```python
from build123d import *

# Parameters (mm, degrees)
SKETCH1_W           = 65.079845806
SKETCH1_H           = 55
SKETCH1_R           = 4
BOSS_EXTRUDE1_DEPTH = 3
SKETCH2_R           = 1
CUT_EXTRUDE1_DEPTH  = 3
FILLET1_R           = 0.5
SKETCH3_R           = 1
CUT_EXTRUDE2_DEPTH  = 52.961426281


with BuildPart() as part:
    # Sketch1 → Boss-Extrude1 (new body)
    with BuildSketch(Plane(origin=(0, 548.352995908, 0), x_dir=(1, 0, 0), z_dir=(0, 1, 0))):
        with Locations((-11.445754552, 0)):
            Rectangle(SKETCH1_W, SKETCH1_H)
        with Locations(Location((0, 0, 0), (0, 0, 270))):
            Circle(SKETCH1_R, mode=Mode.SUBTRACT)
    extrude(amount=BOSS_EXTRUDE1_DEPTH)

    # Sketch2 → Cut-Extrude1 (cut)
    with BuildSketch(Plane(origin=(0, 551.352995908, 0), x_dir=(1, 0, 0), z_dir=(0, 1, 0))):
        with Locations(Location((0, 8, 0), (0, 0, 270))):
            Circle(SKETCH2_R)
        with Locations(Location((5.656854249, 5.656854249, 0), (0, 0, 270))):
            Circle(SKETCH2_R)
        with Locations(Location((8, 0, 0), (0, 0, 270))):
            Circle(SKETCH2_R)
        with Locations(Location((5.656854249, -5.656854249, 0), (0, 0, 270))):
            Circle(SKETCH2_R)
        with Locations(Location((0, -8, 0), (0, 0, 270))):
            Circle(SKETCH2_R)
        with Locations(Location((-5.656854249, -5.656854249, 0), (0, 0, 270))):
            Circle(SKETCH2_R)
        with Locations(Location((-8, 0, 0), (0, 0, 270))):
            Circle(SKETCH2_R)
        with Locations(Location((-5.656854249, 5.656854249, 0), (0, 0, 270))):
            Circle(SKETCH2_R)
    extrude(amount=-CUT_EXTRUDE1_DEPTH, mode=Mode.SUBTRACT)

    # Fillet1
    fillet1_edges = [part.edges().sort_by_distance(p)[0] for p in [
        (21.094168351, 551.352995908, 0),
        (-11.445754552, 551.352995908, -27.5),
        (-43.985677455, 551.352995908, 0),
        (-11.445754552, 548.352995908, -27.5),
        (21.094168351, 548.352995908, 0),
        (-11.445754552, 548.352995908, 27.5),
        (-43.985677455, 548.352995908, 0),
        (-43.985677455, 549.852995908, -27.5),
        (21.094168351, 549.852995908, -27.5),
        (21.094168351, 549.852995908, 27.5),
        (-43.985677455, 549.852995908, 27.5),
        (-11.445754552, 551.352995908, 27.5),
    ]]
    fillet(fillet1_edges, radius=FILLET1_R)

    # Sketch3 → Cut-Extrude2 (cut, through all)
    with BuildSketch(Plane(origin=(0, 551.352995908, 0), x_dir=(1, 0, 0), z_dir=(0, 1, 0))):
        with Locations(Location((-33.485677455, -24, 0), (0, 0, 270))):
            Circle(SKETCH3_R)
        with Locations(Location((-23.485677455, -24, 0), (0, 0, 270))):
            Circle(SKETCH3_R)
        with Locations(Location((16.514322545, -12, 0), (0, 0, 270))):
            Circle(SKETCH3_R)
        with Locations(Location((16.514322545, 12, 0), (0, 0, 270))):
            Circle(SKETCH3_R)
        with Locations(Location((-23.485677455, 24, 0), (0, 0, 270))):
            Circle(SKETCH3_R)
        with Locations(Location((-33.485677455, 24, 0), (0, 0, 270))):
            Circle(SKETCH3_R)
    extrude(amount=-CUT_EXTRUDE2_DEPTH, mode=Mode.SUBTRACT)


solid = part.part
```
Here's how the part is built. I have some questions about the finished solid (model axes, mm). Round coordinates to 2 decimals unless told otherwise and drop trailing zeros. Order: outer loops, then holes, each group sorted by start corner. A loop starts at its lowest first (then second) coordinate and runs counter-clockwise, first axis right, second up. Notation, with made-up numbers: (-28, 75) -> (-14, 75) arc R26 cw to (-14, 102) -> close; hole circle Ø2 at (19, 17). An arc over 180 degrees is marked (long way). Use a Markdown table: item, result. Add a question column.
(1) I need wall thicknesses on line 1 along Z through (x, y) = (-33.5, 549); line 2 along X through (y, z) = (550.5, 0); line 3 along X through (y, z) = (549.45, -5.5). Which ranges of each line are inside material? Lowest first, please.
(2) If we mould it in two halves opening along Z, with no side actions, what happens to faces 1 (the face through (-5.613, 549.874, -6.656)), 2 (the face through (-12, 550, -27.5)), 3 (the face through (-43.986, 550, 0)), 4 (the face through (-12, 550, 27.5))? For each: released by +Z, released by -Z, zero draft, split by the parting line, or undercut.
(3) Suppose I cut it at B-B, the plane z = -12. Please give me the cut outline in (x, y), and give its area (3 significant figures).
(4) For pin 1 Ø1.2 at (x, z) = (-5.66, -5.66) entering from -Y, with a flat end and sliding along its axis, tell me the tip position at first contact or that it passes through.
(5) Suppose I cut it at C-C, the plane z = 0. Please give me the cut outline in (x, y).
(6) Suppose I cut it at A-A, the plane x = 8. Please give me the cut outline in (y, z), and give its area (3 significant figures).
(7) Suppose I cut it at D-D, the plane z = -24. Please give me the cut outline in (x, y).
Verdict:
| question | item | result |
|---|---|---|
| 1 | line 1 | -27.5 to -25, -23 to 23, 25 to 27.5 |
| 1 | line 2 | -43.99 to -9, -7 to -4, 4 to 7, 9 to 21.09 |
| 1 | line 3 | -43.99 to -6.64, -4.67 to 4.67, 6.64 to 21.09 |
| 2 | face 1 | undercut |
| 2 | face 2 | released by -Z |
| 2 | face 3 | zero draft |
| 2 | face 4 | released by +Z |
| 3 | outline | (-43.99, 548.85) arc R0.5 ccw to (-43.49, 548.35) -> (15.51, 548.35) -> (15.51, 551.35) -> (-43.49, 551.35) arc R0.5 ccw to (-43.99, 550.85) -> close; (17.51, 548.35) -> (20.59, 548.35) arc R0.5 ccw to (21.09, 548.85) -> (21.09, 550.85) arc R0.5 ccw to (20.59, 551.35) -> (17.51, 551.35) -> close |
| 3 | area | 189 mm2 |
| 4 | pin 1 | through |
| 5 | outline | (-43.99, 548.85) arc R0.5 ccw to (-43.49, 548.35) -> (-9, 548.35) -> (-9, 551.35) -> (-43.49, 551.35) arc R0.5 ccw to (-43.99, 550.85) -> close; (-7, 548.35) -> (-4, 548.35) -> (-4, 551.35) -> (-7, 551.35) -> close; (4, 548.35) -> (7, 548.35) -> (7, 551.35) -> (4, 551.35) -> close; (9, 548.35) -> (20.59, 548.35) arc R0.5 ccw to (21.09, 548.85) -> (21.09, 550.85) arc R0.5 ccw to (20.59, 551.35) -> (9, 551.35) -> close |
| 6 | outline | (548.35, -27) arc R0.5 ccw to (548.85, -27.5) -> (550.85, -27.5) arc R0.5 ccw to (551.35, -27) -> (551.35, -1) -> (548.35, -1) -> close; (548.35, 1) -> (551.35, 1) -> (551.35, 27) arc R0.5 ccw to (550.85, 27.5) -> (548.85, 27.5) arc R0.5 ccw to (548.35, 27) -> close |
| 6 | area | 159 mm2 |
| 7 | outline | (-43.99, 548.85) arc R0.5 ccw to (-43.49, 548.35) -> (-34.49, 548.35) -> (-34.49, 551.35) -> (-43.49, 551.35) arc R0.5 ccw to (-43.99, 550.85) -> close; (-32.49, 548.35) -> (-24.49, 548.35) -> (-24.49, 551.35) -> (-32.49, 551.35) -> close; (-22.49, 548.35) -> (20.59, 548.35) arc R0.5 ccw to (21.09, 548.85) -> (21.09, 550.85) arc R0.5 ccw to (20.59, 551.35) -> (-22.49, 551.35) -> close |
